```python
from build123d import *

# Parameters (mm, degrees)
SKETCH2_R               = 2.38125
CUT_EXTRUDE3_DEPTH      = 79.994
SKETCH3_R               = 2.38125
CUT_EXTRUDE4_DEPTH      = 67.9290001
CUT_EXTRUDE4_DEPTH_BACK = 67.9290001


with BuildPart() as part:
    # Sketch1 → Revolve1 (revolve)
    with BuildSketch(Plane.XY):
        with BuildLine():
            Line((-78.994, -66.929), (-19.558, -66.929))
            add(Edge.make_bspline(
                [(-19.558, -66.929), (0, -66.929), (0, 0)],
                knots=[3.141592654, 3.141592654, 3.141592654, 4.71238898, 4.71238898, 4.71238898], degree=2, weights=[1, 0.707106781, 1]))
            Line((0, 0), (-9.8933, 0))
            add(Edge.make_bspline(
                [(-19.558, -57.0357), (-9.8933, -57.0357), (-9.8933, 0)],
                knots=[0, 0, 0, 1.570796327, 1.570796327, 1.570796327], degree=2, weights=[1, 0.707106781, 1]))
            Line((-19.558, -57.0357), (-78.994, -57.3786))
            Line((-78.994, -57.3786), (-78.994, -66.929))
        make_face()
    revolve(axis=Axis((-78.994, 0, 0), (1, 0, 0)))

    # Sketch2 → Cut-Extrude3 (cut, through all)
    with BuildSketch(Plane(origin=(0, 0, 0), x_dir=(0, 0, -1), z_dir=(1, 0, 0))):
        with Locations((-25.4, 0)):
            Circle(SKETCH2_R)
        with Locations((25.4, 0)):
            Circle(SKETCH2_R)
    extrude(amount=-CUT_EXTRUDE3_DEPTH, mode=Mode.SUBTRACT)

    # Sketch3 → Cut-Extrude4 (cut, two sides)
    with BuildSketch(Plane.XY) as cut_extrude4_sk:
        with Locations((-25.4, 0)):
            Circle(SKETCH3_R)
    extrude(amount=CUT_EXTRUDE4_DEPTH, mode=Mode.SUBTRACT)
    extrude(cut_extrude4_sk.sketch, amount=-CUT_EXTRUDE4_DEPTH_BACK, mode=Mode.SUBTRACT)


solid = part.part
```
Work out the finished part from the listing and answer in its coordinate system (mm). A direction names the side the tool comes from. Give positions to 0.01 mm unless a question says otherwise; leave off trailing zeros. Order: outer loops, then holes, each group sorted by start corner. A loop starts at its lowest first (then second) coordinate and runs counter-clockwise, first axis right, second up. Notation, with made-up numbers: (82.5, 23.5) - (96.5, 23.5) arc R33 cw to (96.5, 59.5) - close; hole circle Ø3 at (-3.75, 69.5). An arc over 180 degrees is marked (long way). One line per item, written item: value. Start each with the question number.
1. Consider line 1 (Z direction, x = -50.5, y = 0.5); line 2 (X direction, y = 0, z = -63); line 3 (Y direction, x = -25, z = 59). Determine where each line is inside the solid, lowest interval first.
2. Section B-B, the plane x = -72.5 is taken. Write down the section's boundary in (y, z).
3. Section A-A, the plane x = -25.4 is taken. Write down the section's boundary in (y, z), then the cut area to 3 significant figures.
4. Which of the six approach directions +Z, -Z, +X, -X, +Y, -Y give full straight-line access (tool end or side, diameter ignored) to faces 1 (the face through (-27.78, 0.1, -61.9)), 2 (the face through (-49.692, -52.847, 21.912))?
5. Section D-D, the plane x = -56.5 is taken. Write down the section's boundary in (y, z).
6. Section C-C, the plane y = 0 is taken. Count the separate pieces of the cut face and the enclosed holes in it, then the cut area to 3 significant figures.
7. Each of these flat-tipped pins is pushed along its axis until it touches: pin 1 Ø1.5 at (x, z) = (-47, -25) entering from +Y; pin 2 Ø8 at (x, y) = (-45.5, -18) entering from -Z; pin 3 Ø10 at (x, y) = (-22, -42.5) entering from +Z; pin 4 Ø3 at (y, z) = (0, -25.4) entering from -X. Where does it stop, or does it pass through?
8. For a pull along Y with two mould halves and no side action, classify faces 3 (the face through (-6.09, 0.72, 23.13)), 4 (the face through (-78.994, 49.3, -30.1)), 5 (the face through (-48.86, -63.84, -20.1)) as released by +Y, released by -Y, zero draft, split by the parting line, or undercut.
Filled sheet:
1. line 1: -66.93 to -57.21, 57.21 to 66.93
1. line 2: -78.99 to -27.78, -23.02 to -12.96
1. line 3: -31.6 to -2.35, 2.35 to 31.6
2. outline: circle Ø133.86 at (0, 0); hole circle Ø114.68 at (0, 0)
3. outline: (-2.38, -66.89) - (-2.38, -57.02) arc R57.07 cw to (-2.38, 57.02) - (-2.38, 66.89) arc R66.93 ccw to start; (2.38, -66.89) arc R66.93 ccw to (2.38, 66.89) - (2.38, 57.02) arc R57.07 cw to (2.38, -57.02) - close
3. area: 3,750 mm²
4. face 1: +Z, -Z
4. face 2: -X
5. outline: circle Ø133.86 at (0, 0); hole circle Ø114.5 at (0, 0)
6. separate pieces: 5
6. enclosed holes: 0
6. area: 2,160 mm²
7. pin 1: y = 62.38
7. pin 2: z = -65.45
7. pin 3: z = 55.44
7. pin 4: through
8. face 3: undercut
8. face 4: zero draft
8. face 5: split by the parting line
